Check sheet for the modelled part. Datum: model origin and axes. Units: mm. A direction names the side the tool comes from. Round coordinates to 2 decimals unless told otherwise and drop trailing zeros. Write each loop counter-clockwise with the first axis right and the second up, starting at its lowest first coordinate (ties: lowest second). Pieces come first, ordered by that corner, then holes. Notation, with made-up numbers: (-1, 24) -> (3, 24) arc R20 cw to (3, 28) -> close; hole circle Ø11 at (32.25, 84.5). An arc over 180 degrees is marked (long way). One line per item, written item: value.
from build123d import *

# Parameters (mm, degrees)
SKETCH1_W           = 25
SKETCH1_H           = 8.15
SKETCH1_R           = 2.1
BOSS_EXTRUDE1_DEPTH = 5
BOSS_EXTRUDE3_DEPTH = 5
FILLET1_R           = 2.5
SKETCH4_R           = 2.1
BOSS_EXTRUDE4_DEPTH = 5
CUT_EXTRUDE1_DEPTH  = 5
FILLET2_R           = 2.5


with BuildPart() as part:
    # Sketch1 → Boss-Extrude1 (new body)
    with BuildSketch(Plane(origin=(0, 0, 0), x_dir=(1, 0, 0), z_dir=(0, 1, 0))):
        with Locations((8, -0.925)):
            Rectangle(SKETCH1_W, SKETCH1_H)
        with Locations(Location((16, 0, 0), (0, 0, 270))):
            Circle(SKETCH1_R, mode=Mode.SUBTRACT)
        with Locations(Location((0, 0, 0), (0, 0, 270))):
            Circle(SKETCH1_R, mode=Mode.SUBTRACT)
    extrude(amount=BOSS_EXTRUDE1_DEPTH)

    # Sketch3 → Boss-Extrude3 (add)
    with BuildSketch(Plane(origin=(0, 0, -3.15), x_dir=(-1, 0, 0), z_dir=(0, 0, -1))):
        with BuildLine():
            Line((-20.5, 5), (4.5, 5))
            Line((4.5, 5), (4.5, 0))
            Line((4.5, 0), (-8.5, -33.101126286))
            Line((-8.5, -33.101126286), (-8.5, -39.18452209))
            ThreePointArc((-8.5, -39.18452209), (-13.5, -44.18452209), (-18.5, -39.18452209))
            Line((-18.5, -39.18452209), (-18.5, -37.18452209))
            Line((-18.5, -37.18452209), (-40.5, -37.18452209))
            Line((-40.5, -37.18452209), (-40.5, -39.18452209))
            ThreePointArc((-40.5, -39.18452209), (-45.5, -44.18452209), (-50.5, -39.18452209))
            Line((-50.5, -39.18452209), (-50.5, -25.18452209))
            ThreePointArc((-50.5, -25.18452209), (-45.5, -20.18452209), (-40.5, -25.18452209))
            Line((-40.5, -25.18452209), (-40.5, -27.18452209))
            Line((-40.5, -27.18452209), (-31.083364815, -27.18452209))
            Line((-31.083364815, -27.18452209), (-20.5, 0))
            Line((-20.5, 0), (-20.5, 5))
        make_face()
        with BuildLine():
            Line((-6.051156406, -4.816080861), (-15.253856658, -4.816080861))
            Line((-15.253856658, -4.816080861), (-24.092524325, -27.18452209))
            Line((-24.092524325, -27.18452209), (-18.5, -27.18452209))
            Line((-18.5, -27.18452209), (-18.5, -25.18452209))
            ThreePointArc((-18.5, -25.18452209), (-15.76759292, -20.728287991), (-10.55679106, -21.142552133))
            Line((-10.55679106, -21.142552133), (-4.105547887, -4.816080861))
            Line((-4.105547887, -4.816080861), (-6.051156406, -4.816080861))
        make_face(mode=Mode.SUBTRACT)
        with BuildLine():
            Line((-15.6, -39.18452209), (-15.6, -25.18452209))
            ThreePointArc((-15.6, -25.18452209), (-13.5, -23.08452209), (-11.4, -25.18452209))
            Line((-11.4, -25.18452209), (-11.4, -39.18452209))
            ThreePointArc((-11.4, -39.18452209), (-13.5, -41.28452209), (-15.6, -39.18452209))
        make_face(mode=Mode.SUBTRACT)
        with BuildLine():
            Line((-43.4, -25.18452209), (-43.4, -39.18452209))
            ThreePointArc((-43.4, -39.18452209), (-45.5, -41.28452209), (-47.6, -39.18452209))
            Line((-47.6, -39.18452209), (-47.6, -25.18452209))
            ThreePointArc((-47.6, -25.18452209), (-45.5, -23.08452209), (-43.4, -25.18452209))
        make_face(mode=Mode.SUBTRACT)
    extrude(amount=BOSS_EXTRUDE3_DEPTH)

    # Fillet1
    fillet1_edges = [part.edges().sort_by_distance(p)[0] for p in [
        (-4.5, 2.5, 5),
        (20.5, 2.5, 5),
        (31.083364815, -27.18452209, -5.65),
        (24.092524325, -27.18452209, -5.65),
        (15.253856658, -4.816080861, -5.65),
        (40.5, -27.18452209, -5.65),
        (8.5, -33.101126286, -5.65),
        (40.5, -37.18452209, -5.65),
        (18.5, -37.18452209, -5.65),
    ]]
    fillet(fillet1_edges, radius=FILLET1_R)

    # Sketch4 → Boss-Extrude4 (add)
    # profile 1 of 3: a face of its own
    with BuildSketch(Plane(origin=(0, 5, 0), x_dir=(1, 0, 0), z_dir=(0, 1, 0))):
        with BuildLine():
            ThreePointArc((20.5, -2.5), (19.767766953, -4.267766953), (18, -5))
            Line((18, -5), (32.792852268, -5))
            Line((32.792852268, -5), (32.792852268, 8.15))
            Line((32.792852268, 8.15), (20.5, 8.15))
            Line((20.5, 8.15), (20.5, -2.5))
        make_face()
    # profile 2 of 3: a face of its own
    with BuildSketch(Plane(origin=(0, 5, 0), x_dir=(1, 0, 0), z_dir=(0, 1, 0))):
        with BuildLine():
            Line((-2, -5), (18, -5))
            Line((18, -5), (18, -0.640312424))
            ThreePointArc((18, -0.640312424), (13.9, 0), (18, 0.640312424))
            Line((18, 0.640312424), (18, 8.15))
            Line((18, 8.15), (-4.5, 8.15))
            Line((-4.5, 8.15), (-4.5, -2.5))
            ThreePointArc((-4.5, -2.5), (-3.767766953, -4.267766953), (-2, -5))
        make_face()
        with Locations(Location((0, 0, 0), (0, 0, 270))):
            Circle(SKETCH4_R, mode=Mode.SUBTRACT)
    # profile 3 of 3: a face of its own
    with BuildSketch(Plane(origin=(0, 5, 0), x_dir=(1, 0, 0), z_dir=(0, 1, 0))):
        with BuildLine():
            Line((-17.207147732, -5), (-2, -5))
            ThreePointArc((-2, -5), (-3.767766953, -4.267766953), (-4.5, -2.5))
            Line((-4.5, -2.5), (-4.5, 8.15))
            Line((-4.5, 8.15), (-17.207147732, 8.15))
            Line((-17.207147732, 8.15), (-17.207147732, -5))
        make_face()
    extrude(amount=-BOSS_EXTRUDE4_DEPTH)

    # Sketch5 → Cut-Extrude1 (cut)
    with BuildSketch(Plane(origin=(0, 5, 0), x_dir=(1, 0, 0), z_dir=(0, 1, 0))):
        with BuildLine():
            Line((-12, 2.1), (28, 2.1))
            ThreePointArc((28, 2.1), (30.1, 0), (28, -2.1))
            Line((28, -2.1), (-12, -2.1))
            ThreePointArc((-12, -2.1), (-14.1, 0), (-12, 2.1))
        make_face()
    extrude(amount=-CUT_EXTRUDE1_DEPTH, mode=Mode.SUBTRACT)

    # Fillet2
    fillet2_edges = [part.edges().sort_by_distance(p)[0] for p in [
        (32.792852268, 2.5, 5),
        (32.792852268, 2.5, -8.15),
        (-17.207147732, 2.5, 5),
        (-17.207147732, 2.5, -8.15),
    ]]
    fillet(fillet2_edges, radius=FILLET2_R)


solid = part.part
Item 1: Sectioned sample at B-B (z = 0). Enter the section's corners in (x, y).
Result set:
outline: (-17.21, 0) -> (-14.1, 0) -> (-14.1, 5) -> (-17.21, 5) -> close; (30.1, 0) -> (32.79, 0) -> (32.79, 5) -> (30.1, 5) -> close
Item 2: Sectioned sample at A-A (x = 45.5). Enter the section's corners in (y, z), then the cut area to 3 significant figures.
Result set:
outline: (-44.18, -8.15) -> (-41.28, -8.15) -> (-41.28, -3.15) -> (-44.18, -3.15) -> close; (-23.08, -8.15) -> (-20.18, -8.15) -> (-20.18, -3.15) -> (-23.08, -3.15) -> close
area: 29.0 mm^2
Item 3: Tool access check on faces 1 (the cylindrical face through (22.464, -26.118, -5.685)), 2 (the flat face through (8.5, -36, -6)), 3 (the flat face through (29, -37.185, -6)), 4 (the flat face through (32.793, 3, -2)), 5 (the cylindrical face through (30.1, 2.5, 0)). Record the directions out of +Z, -Z, +X, -X, +Y, -Y that give a thin tool (end or side, any length) a straight path to the whole face; none if there is none.
Result set:
face 1: +Z, -Z
face 2: +Z, -Z, -X, -Y
face 3: +Z, -Z, -Y
face 4: +Z, -Z, +X, +Y
face 5: +Y, -Y
Item 4: Depth check by flat-ended pin: pin 1 (4 mm diameter, centred on y = -32, z = -4.5, fed in from -X); pin 2 (5.5 mm diameter, centred on x = 30, z = -4.5, fed in from -Y); pin 3 (2.5 mm diameter, centred on y = -35.5, z = -5.5, fed in from -X). Enter the tip coordinate at first touch or a pass-through.
Result set:
pin 1: x = 7.28
pin 2: y = -37.18
pin 3: x = 8.5
Item 5: Sectioned sample at D-D (y = -29.5). Enter the section's corners in (x, z).
Result set:
outline: (7.09, -8.15) -> (11.4, -8.15) -> (11.4, -3.15) -> (7.09, -3.15) -> close; (15.6, -8.15) -> (43.4, -8.15) -> (43.4, -3.15) -> (15.6, -3.15) -> close; (47.6, -8.15) -> (50.5, -8.15) -> (50.5, -3.15) -> (47.6, -3.15) -> close
Item 6: Material ranges on line 1 along X through (y, z) = (-22, -6.25); line 2 along Z through (x, y) = (16.5, 0.5); line 3 along Z through (x, y) = (17, -1), recorded low to high.
Result set:
line 1: 4.14 to 17.35, 22.04 to 29.06, 41.65 to 49.35
line 2: -8.15 to -2.1, 2.1 to 5
line 3: -8.15 to -3.15
Item 7: Release check for a two-part mould opening along Z. For faces 6 (the flat face through (7.376, -13.094, -5.615)), 7 (the cylindrical face through (32.04, 2.46, 4.29)), 8 (the cylindrical face through (-14.1, 2.5, 0)) record: pulls with the +Z half, pulls with the -Z half, needs draft (parallel to the pull), parting line crosses it, or undercut.
Result set:
face 6: needs draft
face 7: pulls with the +Z half
face 8: undercut
Item 8: Sectioned sample at C-C (x = 6.5). Enter the section's corners in (y, z), then the cut area to 3 significant figures.
Result set:
outline: (-28.01, -8.15) -> (-10.88, -8.15) -> (-10.88, -3.15) -> (-28.01, -3.15) -> close; (-4.82, -8.15) -> (5, -8.15) -> (5, -2.1) -> (0, -2.1) -> (0, -3.15) -> (-4.82, -3.15) -> close; (0, 2.1) -> (5, 2.1) -> (5, 5) -> (0, 5) -> close
area: 154 mm^2
